```python
from build123d import *

# Parameters (mm, degrees)
BOSS_EXTRUDE1_DEPTH = 3.81
FILLET1_R           = 20.32
FILLET3_R           = 25.4
CUT_EXTRUDE8_DEPTH  = 251.19
FILLET4_R           = 20.32
FILLET5_R           = 20.32


with BuildPart() as part:
    # Sketch1 → Boss-Extrude1 (new body)
    with BuildSketch(Plane.XY):
        Polygon((0, 76.2), (38.1, 101.6), (190.5, 101.6), (228.6, 76.2), (228.6, 0), (0, 0), align=None)
    extrude(amount=BOSS_EXTRUDE1_DEPTH)

    # Fillet1
    fillet1_edges = [part.edges().sort_by_distance(p)[0] for p in [
        (190.5, 101.6, 1.905),
        (38.1, 101.6, 1.905),
    ]]
    fillet(fillet1_edges, radius=FILLET1_R)

    # Fillet3
    fillet3_edges = [part.edges().sort_by_distance(p)[0] for p in [
        (0, 76.2, 1.905),
        (228.6, 76.2, 1.905),
    ]]
    fillet(fillet3_edges, radius=FILLET3_R)

    # Sketch2 → Cut-Extrude8 (cut, through all)
    with BuildSketch(Plane.XY.offset(3.81)):
        with BuildLine():
            Line((72.324780666, 0), (0, 0))
            Line((0, 0), (0, 32.483690967))
            add(Edge.make_bspline(
                [(0, 32.483690967), (10.059478489, 1.840398762), (47.836090043, 3.417036799), (72.324780666, 0)],
                knots=[0, 0, 0, 0, 1, 1, 1, 1], degree=3))
        make_face()
        with BuildLine():
            Line((156.275219334, 0), (228.6, 0))
            Line((228.6, 0), (228.6, 32.483690967))
            add(Edge.make_bspline(
                [(228.6, 32.483690967), (218.540521511, 1.840398762), (180.763909957, 3.417036799), (156.275219334, 0)],
                knots=[0, 0, 0, 0, 1, 1, 1, 1], degree=3))
        make_face()
    extrude(amount=-CUT_EXTRUDE8_DEPTH, mode=Mode.SUBTRACT)

    # Fillet4
    fillet4_edges = [part.edges().sort_by_distance(p)[0] for p in [
        (0, 32.483690967, 1.905),
        (228.6, 32.483690967, 1.905),
    ]]
    fillet(fillet4_edges, radius=FILLET4_R)

    # Fillet5
    fillet5_edges = [part.edges().sort_by_distance(p)[0] for p in [
        (72.324780666, 0, 1.905),
        (156.275219334, 0, 1.905),
    ]]
    fillet(fillet5_edges, radius=FILLET5_R)


solid = part.part
```
Verification items for the finished model (mm, model axes). Give positions to 0.01 mm unless a question says otherwise; leave off trailing zeros. Return JSON: item names as keys, results as strings. Group by question number.
1) Mould release check, pull along Z, two halves, no side actions. Record for faces 1 (the face through (116, 52, 3.81)), 2 (the face through (21.99, 90.86, 1.88)), 3 (the face through (116, 52, 0)): pulls with the +Z half, pulls with the -Z half, needs draft (parallel to the pull), parting line crosses it, or undercut.
2) Go/stop test with flat-tipped pins: pin 1 Ø2 at (x, z) = (41.5, 3) entering from +Y; pin 2 Ø2 at (y, z) = (34.5, 3) entering from +X. Record where each tip stops, or that it passes through.
3) Scan lines: line 1 (X direction, y = 36, z = 2.8); line 2 (X direction, y = 77.5, z = 2.05); line 3 (Y direction, x = 72, z = 1.5). Record each from-to range of solid material in increasing order.
Answer block:
{
 "1": {"face 1": "pulls with the +Z half", "face 2": "needs draft", "face 3": "pulls with the -Z half"},
 "2": {"pin 1": "stops at y = 101.52", "pin 2": "stops at x = 228.58"},
 "3": {"line 1": "x = 0 to 228.6", "line 2": "x = 4.82 to 223.78", "line 3": "y = 0.07 to 101.6"}
}
